Here's the drawing with two shaded views (mm, measured from the low corner). I have some questions. A direction names the side the tool comes from. Give positions to 0.01 mm unless a question says otherwise; leave off trailing zeros. Order: outer loops, then holes, each group sorted by start corner. A loop starts at its lowest first (then second) coordinate and runs counter-clockwise, first axis right, second up. Notation, with made-up numbers: M 58,48 L 65,48 A9 ccw 65,64 Z; hole C -27.75,88 d5. An arc over 180 degrees is marked long. Use a Markdown table: item, result. Add a question column.
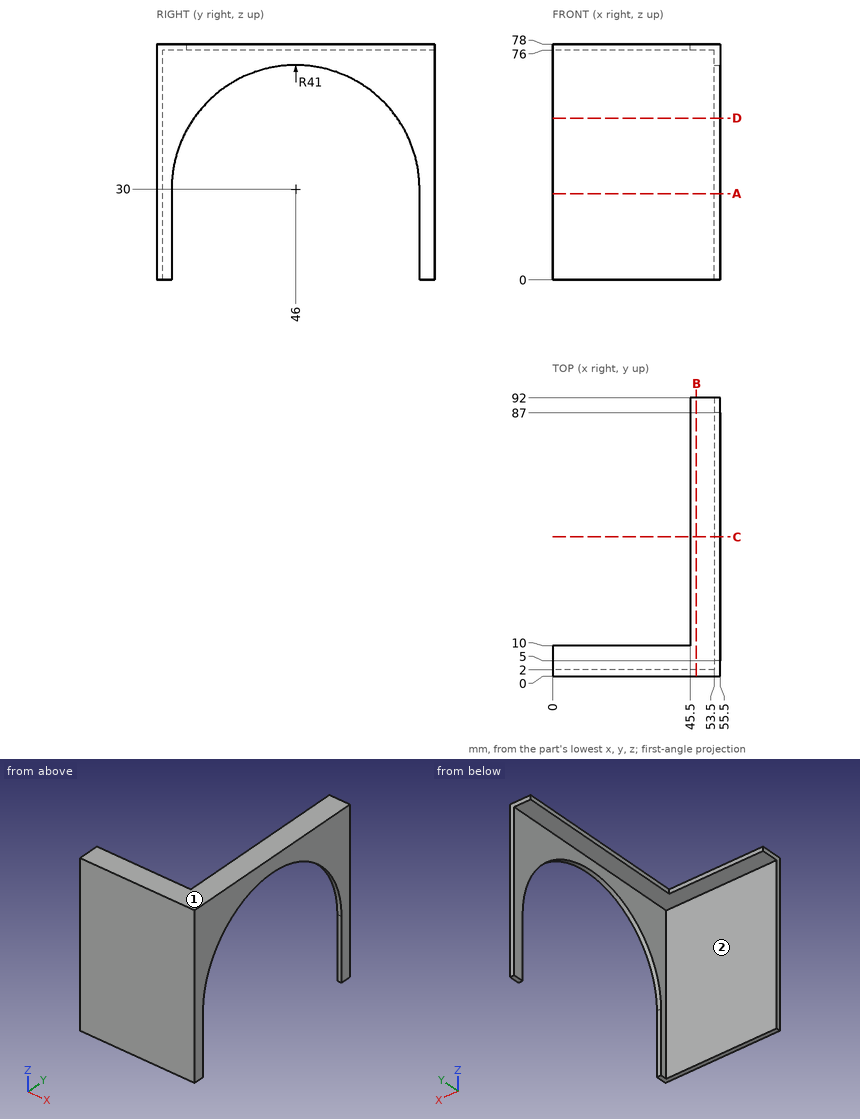
1. I need wall thicknesses on L1, parallel to Y at x = 20.5, z = 72.5; L2, parallel to Z at x = 3, y = 8.5. Which ranges of each line are inside material? Lowest first, please. Write a range as [from, to].
2. Will these pins go through, and if not, where does the flat tip stop? pin 1 (3 mm diameter, centred on x = 39.5, z = 31.5, fed in from +Y); pin 2 (2 mm diameter, centred on x = 29.5, z = 76.5, fed in from +Y); pin 3 (1 mm diameter, centred on y = 39, z = 76.5, fed in from -X).
3. If we section it at B-B, the plane x = 47.5: List the corners of the cut face in (y, z) for me.
4. On a 3-axis mill with a long thin cutter (end or side, diameter ignored), from which of +Z, -Z, +X, -X, +Y, -Y can I reach the whole of each face in a straight line? I mean the marked faces 1 and 2. Say none if no direction works.
5. If we section it at C-C, the plane y = 46: List the corners of the cut face in (x, z) for me, then the cut area to 3 significant figures.
6. If we section it at A-A, the plane z = 28.5: List the corners of the cut face in (x, y) for me.
7. If we section it at D-D, the plane z = 53.5: List the corners of the cut face in (x, y) for me.
Geometry results:
| question | item | result |
|---|---|---|
| 1 | L1 | y = [0, 2] |
| 1 | L2 | z = [76, 78] |
| 2 | pin 1 | stops at y = 2 |
| 2 | pin 2 | stops at y = 10 |
| 2 | pin 3 | stops at x = 45.5 |
| 3 | outline | M 0,0 L 2,0 L 2,76 L 92,76 L 92,78 L 0,78 Z |
| 4 | face 1 | +Z, +X, -X, +Y, -Y |
| 4 | face 2 | -Z, -X, +Y |
| 5 | outline | M 45.5,76 L 53.5,76 L 53.5,71 L 55.5,71 L 55.5,78 L 45.5,78 Z |
| 5 | area | 30.0 mm^2 |
| 6 | outline | M 0,0 L 55.5,0 L 55.5,5 L 53.5,5 L 53.5,2 L 0,2 Z; M 53.5,87 L 55.5,87 L 55.5,92 L 53.5,92 Z |
| 7 | outline | M 0,0 L 55.5,0 L 55.5,12.4 L 53.5,12.4 L 53.5,2 L 0,2 Z; M 53.5,79.6 L 55.5,79.6 L 55.5,92 L 53.5,92 Z |
